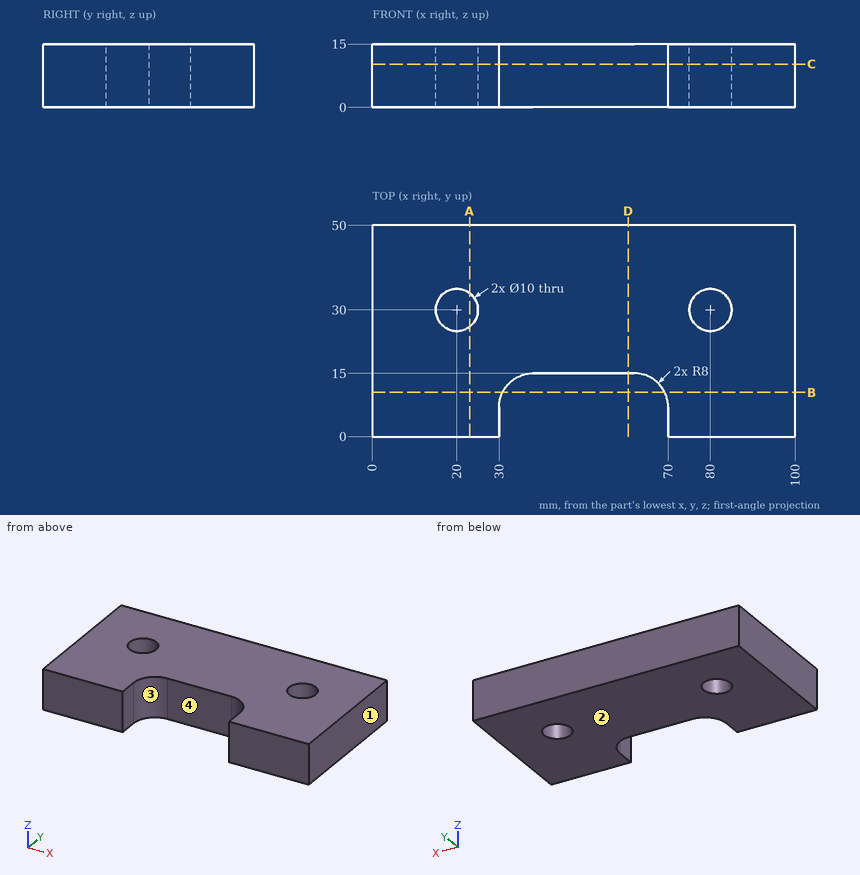
Input: dimensioned drawing with shaded views. Units: mm. Origin: part minimum x, y, z. Give positions to 0.01 mm unless a question says otherwise; leave off trailing zeros. Loops run counter-clockwise (first coordinate to the right, second up) from the corner with the lowest first, then second, coordinate; pieces in that order, holes last. Notation, with made-up numbers: (-24, 84.25) -> (20, 84.25) arc R33 ccw to (20, 121.25) -> close; hole circle Ø9 at (-15.75, 22.25). An arc over 180 degrees is marked (long way). Return JSON: item names as keys, results as strings.
Item 1: Pin query (flat end, axial travel): P1, Ø1, axis at x = 36, z = 4, coming from the -Y side. Return the tip coordinate at first contact, or that it passes through.
Filled in:
{"P1": "y = 14.6"}
Item 2: Mould query, pull axis X, two halves, no side actions, for the marked faces 1, 2, 3 and 4. Classes: released by +X, released by -X, zero draft, split by the parting line, or undercut.
Filled in:
{"face 1": "released by +X", "face 2": "zero draft", "face 3": "undercut", "face 4": "undercut"}
Item 3: Line query: line 1 (X direction, y = 30, z = 11.5); line 2 (Y direction, x = 80, z = 5.75); line 3 (X direction, y = 33, z = 9.75). Output: solid intervals per line, ascending.
Filled in:
{"line 1": "0 to 15, 25 to 75, 85 to 100", "line 2": "0 to 25, 35 to 50", "line 3": "0 to 16, 24 to 76, 84 to 100"}
Item 4: Section B-B, the plane y = 10.5. Output: boundary loops of the cut face in (x, z).
Filled in:
{"outline": "(0, 0) -> (30.81, 0) -> (30.81, 15) -> (0, 15) -> close; (69.19, 0) -> (100, 0) -> (100, 15) -> (69.19, 15) -> close"}
Item 5: Section D-D, the plane x = 60.5. Output: boundary loops of the cut face in (y, z).
Filled in:
{"outline": "(15, 0) -> (50, 0) -> (50, 15) -> (15, 15) -> close"}
Item 6: Section C-C, the plane z = 10.25. Output: boundary loops of the cut face in (x, y), plus the area to 3 significant figures.
Filled in:
{"outline": "(0, 0) -> (30, 0) -> (30, 7) arc R8 cw to (38, 15) -> (62, 15) arc R8 cw to (70, 7) -> (70, 0) -> (100, 0) -> (100, 50) -> (0, 50) -> close; hole circle Ø10 at (20, 30); hole circle Ø10 at (80, 30)", "area": "4,270 mm^2"}
Item 7: Section A-A, the plane x = 23. Output: boundary loops of the cut face in (y, z), plus the area to 3 significant figures.
Filled in:
{"outline": "(0, 0) -> (26, 0) -> (26, 15) -> (0, 15) -> close; (34, 0) -> (50, 0) -> (50, 15) -> (34, 15) -> close", "area": "630 mm^2"}
